from build123d import *

# Parameters (mm, degrees)
F0_W     = 128
F0_H     = 200
F1_DEPTH = 5
F2_R     = 1.25
F2_R_2   = 1.7
F3_DEPTH = 25
F5_DEPTH = 3


with BuildPart() as f1:
    # F0 (on Top) → F1 (new body)
    with BuildSketch(Plane.XY):
        with Locations((64, 100)):
            Rectangle(F0_W, F0_H)
    extrude(amount=F1_DEPTH)

    # F2 (on face) → F3 (cut)
    with BuildSketch(Plane.XY.offset(5)):
        with Locations((113.915, 6)):
            Circle(F2_R)
        with Locations((4, 196)):
            Circle(F2_R_2)
        with Locations((124, 196)):
            Circle(F2_R_2)
        with Locations((4, 4)):
            Circle(F2_R_2)
        with Locations((124, 4)):
            Circle(F2_R_2)
        with Locations((43.915, 6)):
            Circle(F2_R)
        with Locations((85.915, 6)):
            Circle(F2_R)
        with Locations((71.915, 6)):
            Circle(F2_R)
        with Locations((29.915, 6)):
            Circle(F2_R)
        with Locations((15.915, 6)):
            Circle(F2_R)
        with Locations((57.915, 6)):
            Circle(F2_R)
        with Locations((99.915, 6)):
            Circle(F2_R)
    extrude(amount=-F3_DEPTH, mode=Mode.SUBTRACT)

    # F4 (on face) → F5 (cut)
    with BuildSketch(Plane.XY.offset(5)):
        with BuildLine():
            ThreePointArc((119.9, 190), (118.435534, 193.535534), (114.9, 195))
            Line((114.9, 195), (112.7, 195))
            ThreePointArc((112.7, 195), (109.164466, 193.535534), (107.7, 190))
            Line((107.7, 190), (107.7, 30))
            ThreePointArc((107.7, 30), (109.164466, 26.464466), (112.7, 25))
            Line((112.7, 25), (114.9, 25))
            ThreePointArc((114.9, 25), (118.435534, 26.464466), (119.9, 30))
            Line((119.9, 30), (119.9, 190))
        make_face()
        with BuildLine():
            ThreePointArc((105.9, 190), (104.435534, 193.535534), (100.9, 195))
            Line((100.9, 195), (98.7, 195))
            ThreePointArc((98.7, 195), (95.164466, 193.535534), (93.7, 190))
            Line((93.7, 190), (93.7, 30))
            ThreePointArc((93.7, 30), (95.164466, 26.464466), (98.7, 25))
            Line((98.7, 25), (100.9, 25))
            ThreePointArc((100.9, 25), (104.435534, 26.464466), (105.9, 30))
            Line((105.9, 30), (105.9, 190))
        make_face()
        with BuildLine():
            Line((86.9, 195), (84.7, 195))
            ThreePointArc((84.7, 195), (81.164466, 193.535534), (79.7, 190))
            Line((79.7, 190), (79.7, 30))
            ThreePointArc((79.7, 30), (81.164466, 26.464466), (84.7, 25))
            Line((84.7, 25), (86.9, 25))
            ThreePointArc((86.9, 25), (90.435534, 26.464466), (91.9, 30))
            Line((91.9, 30), (91.9, 190))
            ThreePointArc((91.9, 190), (90.435534, 193.535534), (86.9, 195))
        make_face()
        with BuildLine():
            Line((72.9, 195), (70.7, 195))
            ThreePointArc((70.7, 195), (67.164466, 193.535534), (65.7, 190))
            Line((65.7, 190), (65.7, 30))
            ThreePointArc((65.7, 30), (67.164466, 26.464466), (70.7, 25))
            Line((70.7, 25), (72.9, 25))
            ThreePointArc((72.9, 25), (76.435534, 26.464466), (77.9, 30))
            Line((77.9, 30), (77.9, 190))
            ThreePointArc((77.9, 190), (76.435534, 193.535534), (72.9, 195))
        make_face()
        with BuildLine():
            Line((58.9, 195), (56.7, 195))
            ThreePointArc((56.7, 195), (53.164466, 193.535534), (51.7, 190))
            Line((51.7, 190), (51.7, 30))
            ThreePointArc((51.7, 30), (53.164466, 26.464466), (56.7, 25))
            Line((56.7, 25), (58.9, 25))
            ThreePointArc((58.9, 25), (62.435534, 26.464466), (63.9, 30))
            Line((63.9, 30), (63.9, 190))
            ThreePointArc((63.9, 190), (62.435534, 193.535534), (58.9, 195))
        make_face()
        with BuildLine():
            Line((44.9, 195), (42.7, 195))
            ThreePointArc((42.7, 195), (39.164466, 193.535534), (37.7, 190))
            Line((37.7, 190), (37.7, 30))
            ThreePointArc((37.7, 30), (39.164466, 26.464466), (42.7, 25))
            Line((42.7, 25), (44.9, 25))
            ThreePointArc((44.9, 25), (48.435534, 26.464466), (49.9, 30))
            Line((49.9, 30), (49.9, 190))
            ThreePointArc((49.9, 190), (48.435534, 193.535534), (44.9, 195))
        make_face()
        with BuildLine():
            Line((30.9, 195), (28.7, 195))
            ThreePointArc((28.7, 195), (25.164466, 193.535534), (23.7, 190))
            Line((23.7, 190), (23.7, 30))
            ThreePointArc((23.7, 30), (25.164466, 26.464466), (28.7, 25))
            Line((28.7, 25), (30.9, 25))
            ThreePointArc((30.9, 25), (34.435534, 26.464466), (35.9, 30))
            Line((35.9, 30), (35.9, 190))
            ThreePointArc((35.9, 190), (34.435534, 193.535534), (30.9, 195))
        make_face()
        with BuildLine():
            Line((16.9, 195), (14.7, 195))
            ThreePointArc((14.7, 195), (11.164466, 193.535534), (9.7, 190))
            Line((9.7, 190), (9.7, 30))
            ThreePointArc((9.7, 30), (11.164466, 26.464466), (14.7, 25))
            Line((14.7, 25), (16.9, 25))
            ThreePointArc((16.9, 25), (20.435534, 26.464466), (21.9, 30))
            Line((21.9, 30), (21.9, 190))
            ThreePointArc((21.9, 190), (20.435534, 193.535534), (16.9, 195))
        make_face()
    extrude(amount=-F5_DEPTH, mode=Mode.SUBTRACT)


solid = f1.part
Can you work these out from the model? Positions are in its coordinate system, mm. A direction names the side the tool comes from. Coordinates: 2 decimals unless noted, no trailing zeros. Write each loop counter-clockwise with the first axis right and the second up, starting at its lowest first coordinate (ties: lowest second). Pieces come first, ordered by that corner, then holes.
Q1. For P1, Ø6, axis at x = 59.5, y = 123.5, coming from the +Z side, with a flat end and sliding along its axis, tell me the tip position at first contact or that it passes through.
Results found:
P1: stops at z = 2
Q2. Imagine slicing it at A-A, the plane z = 3.85. Count the separate pieces of the cut face and the enclosed holes in it, plus the area to 3 significant figures.
Results found:
separate pieces: 1
enclosed holes: 20
area: 9,100 mm2
Q3. Which directions (+Z, -Z, +X, -X, +Y, -Y) give clear straight access to the entire face, cutting with the end or side of a thin tool? Please do faces 3 (the face through (63, 101, 0)), 4 (the face through (53.13, 26.5, 3.52)).
Results found:
face 3: -Z, +X, -X, +Y, -Y
face 4: +Z
Q4. If we mould it in two halves opening along Y, with no side actions, what happens to faces 1 (the face through (67.2, 193.57, 3.52)), 2 (the face through (128, 99, 2))? For each: +Y half, -Y half, draft (parallel to the pull), parting line (faces both ways), or undercut.
Results found:
face 1: undercut
face 2: draft
Q5. Imagine slicing it at B-B, the plane x = 110.5. List the corners of the cut face in (y, z) for me, plus the area to 3 significant figures.
Results found:
outline: (0, 0) - (200, 0) - (200, 5) - (194.49, 5) - (194.49, 2) - (25.51, 2) - (25.51, 5) - (0, 5) - close
area: 493 mm2
Q6. Please list where these lines run through material, in increasing order: L1, parallel to X at y = 196, z = 3.2; L2, parallel to Y at x = 58.5, z = 2.5; L3, parallel to Z at x = 31, y = 51.5.
Results found:
L1: x = 0 to 2.3, 5.7 to 122.3, 125.7 to 128
L2: y = 0 to 4.9, 7.1 to 25, 195 to 200
L3: z = 0 to 2
